```python
from build123d import *

# Parameters (mm, degrees)
BOSS_EXTRUDE1_DEPTH = 10
BOSS_EXTRUDE2_DEPTH = 10


with BuildPart() as part:
    # Sketch1 → Boss-Extrude1 (new body)
    with BuildSketch(Plane(origin=(0, 0, 0), x_dir=(0, 0, -1), z_dir=(1, 0, 0))):
        with BuildLine():
            Line((-76.592461771, 20.953089015), (1.366493243, 12.273096648))
            ThreePointArc((1.366493243, 12.273096648), (12.345744217, -0.280722022), (0.807229086, -12.322523537))
            Line((0.807229086, -12.322523537), (-77.465686513, -17.45005881))
            ThreePointArc((-77.465686513, -17.45005881), (-98.002496493, 2.228416408), (-76.592461771, 20.953089015))
        make_face()
        with BuildLine():
            Line((-77.661791455, -14.456475197), (0.611124144, -9.328939923))
            ThreePointArc((0.611124144, -9.328939923), (9.339609214, -0.417483589), (1.441037018, 9.237207648))
            Line((1.441037018, 9.237207648), (-76.216477855, 17.876925629))
            ThreePointArc((-76.216477855, 17.876925629), (-94.991237369, 2.517160117), (-77.661791455, -14.456475197))
        make_face(mode=Mode.SUBTRACT)
    extrude(amount=BOSS_EXTRUDE1_DEPTH)

    # Sketch2 → Boss-Extrude2 (add)
    with BuildSketch(Plane.ZY):
        with BuildLine():
            Line((-6.336674596, 0.518546587), (-9.195436771, 1.687167861))
            ThreePointArc((-9.195436771, 1.687167861), (-9.3441708, -0.298437374), (-9.069035243, -2.270504914))
            Line((-9.069035243, -2.270504914), (-6.299160688, -0.86192234))
            Line((-6.299160688, -0.86192234), (-6.336674596, 0.518546587))
        make_face()
    extrude(amount=-BOSS_EXTRUDE2_DEPTH)


solid = part.part
```
Part model, mm, in its own coordinate system. A direction names the side the tool comes from. Coordinates: 2 decimals unless noted, no trailing zeros. Write each loop counter-clockwise with the first axis right and the second up, starting at its lowest first coordinate (ties: lowest second). Pieces come first, ordered by that corner, then holes.
Item 1: Probe line 1 (Y direction, x = 0.75, z = 44.5); line 2 (Z direction, x = 4, y = 7); line 3 (Y direction, x = 4.5, z = 56.5). List the from-to ranges inside material, lowest first.
Item 2: Which spindle directions (+Z, -Z, +X, -X, +Y, -Y) get a long thin tool onto all of the face, cutting with end or side? Do faces 1 (the face through (4.93, -1.576, -7.703)), 2 (the face through (10, 15, 43)). Say none if no direction does.
Item 3: Slice it at C-C (y = 6). Write the cut outline in (x, z), and give its area (3 significant figures).
Item 4: Slice it at B-B (x = 3.5). Write the cut outline in (y, z).
Item 5: Pin check, flat tips, straight feed: pin 1 (6 mm diameter, centred on x = 4, z = 68.5, fed in from -Y); pin 2 (5 mm diameter, centred on y = -12, z = 57.5, fed in from +X); pin 3 (3 mm diameter, centred on x = 1.5, z = 5.5, fed in from +Y); pin 4 (5 mm diameter, centred on x = 8.5, z = 74.5, fed in from +Y). Stop position of each tip, or through.
Item 6: Slice it at A-A (z = 50). Write the cut outline in (x, y), and give its area (3 significant figures).
Results found:
1. line 1: y = -15.29 to -12.28, 14.35 to 17.38
1. line 2: z = -10.17 to -6.2, 94.15 to 97.29
1. line 3: y = -16.08 to -13.07, 15.68 to 18.72
2. face 1: +X, -X
2. face 2: +Z, -Z, +X, +Y, -Y
3. outline: (0, -10.79) - (10, -10.79) - (10, -7.17) - (0, -7.17) - close; (0, 94.45) - (10, 94.45) - (10, 97.54) - (0, 97.54) - close
3. area: 67.1 mm2
4. outline: (-17.45, 77.47) - (-12.32, -0.81) arc R12.35 ccw to (12.27, -1.37) - (20.95, 76.59) arc R19.28 ccw (long way) to start; hole (-14.46, 77.66) - (-9.33, -0.61) arc R9.35 ccw to (-2.27, -9.07) - (-0.86, -6.3) - (0.52, -6.34) - (1.69, -9.2) arc R9.35 ccw to (9.24, -1.44) - (17.88, 76.22) arc R16.28 ccw (long way) to start
5. pin 1: stops at y = -17.06
5. pin 2: stops at x = 10
5. pin 3: stops at y = 13.2
5. pin 4: stops at y = 20.99
6. outline: (0, -15.65) - (10, -15.65) - (10, -12.64) - (0, -12.64) - close; (0, 14.96) - (10, 14.96) - (10, 17.99) - (0, 17.99) - close
6. area: 60.4 mm2
